```python
from build123d import *

# Parameters (mm, degrees)
BOSS_EXTRUDE1_DEPTH      = 10
SKETCH2_OUTSIDE_W        = 47.45
SKETCH2_OUTSIDE_H        = 30.449999999999996
CUT_EXTRUDE1_DEPTH       = 20
F_2_0MM_DOWEL_HOLE1_D    = 2
M3_CLEARANCE_HOLE1_D     = 3.6
M3_CLEARANCE_HOLE1_DEPTH = 4
M3_CLEARANCE_HOLE1_TIP   = 1.0815491142496085
FILLET2_R                = 3
FILLET3_R                = 5
FILLET5_R                = 0.5
CUT_EXTRUDE2_REACH       = 40.536
SKETCH14_W               = 3.6000000000000014
SKETCH14_H               = 4
FILLET6_R                = 1


with BuildPart() as part:
    # Sketch1 → Boss-Extrude1 (new, symmetric)
    with BuildSketch(Plane.XY):
        Polygon((0, 0), (0, 4), (-37, 3.9999999999999956), (-37, 0), align=None)
    extrude(amount=BOSS_EXTRUDE1_DEPTH, both=True)

    # Sketch2 outside → Cut-Extrude1 (cut)
    with BuildSketch(Plane.XZ):
        with Locations((-18.5, 0)):
            Rectangle(SKETCH2_OUTSIDE_W, SKETCH2_OUTSIDE_H)
        with BuildLine():
            Line((-12.7, -7.800000000000001), (-12.699999999999998, 4.7))
            ThreePointArc((-12.699999999999998, 4.7), (-8.944365081389599, 3.144365081389597), (-10.5, 6.899999999999999))
            Line((-10.5, 6.899999999999999), (3.8e-16, 6.9))
            Line((3.8e-16, 6.9), (0, 10))
            Line((0, 10), (-15.699999999999996, 10.000000000000002))
            Line((-15.699999999999996, 10.000000000000002), (-21.733310313031556, -0.449999999999999))
            Line((-21.733310313031556, -0.449999999999999), (-37, -0.4499999999999973))
            Line((-37, -0.4499999999999973), (-37, -8.450000000000001))
            Line((-37, -8.450000000000001), (-21.733310313031556, -8.45))
            Line((-21.733310313031556, -8.45), (-15.699999999999996, -10.000000000000002))
            Line((-15.699999999999996, -10.000000000000002), (-10.499999999999998, -9.999999999999998))
            ThreePointArc((-10.499999999999998, -9.999999999999998), (-8.944365081389593, -6.244365081389596), (-12.7, -7.800000000000001))
        make_face(mode=Mode.SUBTRACT)
    extrude(amount=-CUT_EXTRUDE1_DEPTH, mode=Mode.SUBTRACT)

    # Ø2.0mm Dowel Hole1 (through all)
    with Locations(Plane(origin=(0, 0, 0), x_dir=(-1, 0, 0), z_dir=(0, -1, 0))):
        with Locations((10.5, -4.7), (10.5, 7.8)):
            Hole(F_2_0MM_DOWEL_HOLE1_D / 2)

    # M3 Clearance Hole1
    with Locations(Plane(origin=(0, 0, 0), x_dir=(-1, 0, 0), z_dir=(0, -1, 0))):
        with Locations((32.5, 4.45)):
            Hole(M3_CLEARANCE_HOLE1_D / 2, depth=M3_CLEARANCE_HOLE1_DEPTH)
            with Locations((0, 0, -(M3_CLEARANCE_HOLE1_DEPTH + M3_CLEARANCE_HOLE1_TIP / 2))):  # 118° drill point
                Cone(0, M3_CLEARANCE_HOLE1_D / 2, M3_CLEARANCE_HOLE1_TIP, mode=Mode.SUBTRACT)

    # Fillet2
    fillet2_edges = [part.edges().sort_by_distance(p)[0] for p in [
        (-37, 1.9999999999999978, -0.4499999999999973),
    ]]
    fillet(fillet2_edges, radius=FILLET2_R)

    # Fillet3
    fillet3_edges = [part.edges().sort_by_distance(p)[0] for p in [
        (-15.699999999999996, 1.9999999999999991, 10.000000000000002),
        (-15.699999999999996, 1.9999999999999991, -10.000000000000002),
        (-21.733310313031556, 1.9999999999999987, -0.449999999999999),
        (-21.733310313031556, 1.9999999999999987, -8.45),
    ]]
    fillet(fillet3_edges, radius=FILLET3_R)

    # Fillet5
    fillet5_edges = [part.edges().sort_by_distance(p)[0] for p in [
        (-10.5, 1.9999999999999993, 6.899999999999999),
        (-12.699999999999998, 1.9999999999999993, 4.7),
        (-12.7, 1.9999999999999993, -7.800000000000001),
    ]]
    fillet(fillet5_edges, radius=FILLET5_R)

    # Sketch14 → Cut-Extrude2 (cut, up to next)
    with BuildSketch(Plane.XZ, mode=Mode.PRIVATE) as cut_extrude2_sk1:
        with Locations((-32.5, -6.449999999999999)):
            Rectangle(SKETCH14_W, SKETCH14_H)
    cut_extrude2_tool1 = extrude(cut_extrude2_sk1.sketch, amount=-CUT_EXTRUDE2_REACH, mode=Mode.PRIVATE) & part.part
    add(cut_extrude2_tool1.solids().sort_by_distance((-32.5, 0, -6.45))[0], mode=Mode.SUBTRACT)

    # Fillet6
    fillet6_edges = [part.edges().sort_by_distance(p)[0] for p in [
        (-30.700000000000003, 1.9999999999999982, -8.45),
        (-34.300000000000004, 1.999999999999998, -8.45),
    ]]
    fillet(fillet6_edges, radius=FILLET6_R)

    # Mirror1: part across plane


with BuildPart() as part_1:
    add(part.part)
    add(part.part.mirror(Plane(origin=(0, 0, -10), x_dir=(0, 0, 1), z_dir=(1, 0, 0))))


solid = part_1.part
```
Verification items for the finished model (mm, model axes). A direction names the side the tool comes from. Give positions to 0.01 mm unless a question says otherwise; leave off trailing zeros. Order: outer loops, then holes, each group sorted by start corner. A loop starts at its lowest first (then second) coordinate and runs counter-clockwise, first axis right, second up. Notation, with made-up numbers: (28.25, 34) -> (67.25, 34) arc R31 cw to (67.25, 70) -> close; hole circle Ø3 at (-25, -6). An arc over 180 degrees is marked (long way). One line per item, written item: value.
(1) Draft check along X on faces 4 (the face through (0, 2, 10)), 5 (the face through (30.7, 2, -6)), 6 (the face through (-22.152, 2.028, 0.202)). Enter one of: pulls with the +X half, pulls with the -X half, needs draft (parallel to the pull), parting line crosses it, or undercut.
Final values:
face 4: needs draft
face 5: undercut
face 6: pulls with the -X half
(2) Sectioned sample at B-B on z = 1. Record the cut outline in (x, y).
Final values:
outline: (-21.1, 0) -> (-12.7, 0) -> (-12.7, 4) -> (-21.1, 4) -> close; (12.7, 0) -> (21.1, 0) -> (21.1, 4) -> (12.7, 4) -> close
(3) Sectioned sample at A-A on z = 4.7. Record the cut outline in (x, y).
Final values:
outline: (-18.76, 0) -> (-11.5, 0) -> (-11.5, 4) -> (-18.76, 4) -> close; (-9.5, 0) -> (-8.3, 0) -> (-8.3, 4) -> (-9.5, 4) -> close; (8.3, 0) -> (9.5, 0) -> (9.5, 4) -> (8.3, 4) -> close; (11.5, 0) -> (18.76, 0) -> (18.76, 4) -> (11.5, 4) -> close
(4) Sectioned sample at C-C on x = 27. Record the cut outline in (y, z).
Final values:
outline: (0, -8.45) -> (4, -8.45) -> (4, -0.45) -> (0, -0.45) -> close
(5) Sectioned sample at D-D on z = -1.75. Record the cut outline in (x, y).
Final values:
outline: (-36.47, 0) -> (-12.7, 0) -> (-12.7, 4) -> (-36.47, 4) -> close; (12.7, 0) -> (36.47, 0) -> (36.47, 4) -> (12.7, 4) -> close
(6) Scan lines: line 1 along Z through (x, y) = (10.5, 3.25); line 2 along X through (y, z) = (3.3, -5); line 3 along X through (y, z) = (2.8, -7.8). Record each from-to range of solid material in increasing order. Write a range as [from, to].
Final values:
line 1: [-10, -8.8], [-6.8, -5.6], [2.5, 3.7], [5.7, 10]
line 2: [-37, -34.3], [-30.7, -12.7], [12.7, 30.7], [34.3, 37]
line 3: [-37, -34.36], [-30.64, -11.5], [-9.5, -8.3], [8.3, 9.5], [11.5, 30.64], [34.36, 37]
(7) Gauge pin test, flat ends, axial feed: pin 1 (2 mm diameter, centred on x = -24, z = -4.5, fed in from -Y); pin 2 (1.6 mm diameter, centred on x = -10.5, z = -7.8, fed in from +Y); pin 3 (2 mm diameter, centred on y = 1, z = -1, fed in from -X); pin 4 (0.9 mm diameter, centred on x = -36, y = 2, fed in from -Z). Record the tip position at first contact, or that the pin passes through.
Final values:
pin 1: y = 0
pin 2: through
pin 3: x = -36.63
pin 4: z = -8.45
(8) Tool access check on faces 1 (the face through (36, 2, -8.45)), 2 (the face through (-29, 2, -0.45)), 3 (the face through (12.7, 2, -2)). Record the directions out of +Z, -Z, +X, -X, +Y, -Y that give a thin tool (end or side, any length) a straight path to the whole face; none if there is none.
Final values:
face 1: -Z, +X, +Y, -Y
face 2: +Z, -X, +Y, -Y
face 3: +Y, -Y
